Answer from the drawing. Dimensions are ordinates in mm from the lowest x, y and z of the part. Give positions to 0.01 mm unless a question says otherwise; leave off trailing zeros. Loops run counter-clockwise (first coordinate to the right, second up) from the corner with the lowest first, then second, coordinate; pieces in that order, holes last.
(1) Find section C-C, the plane y = 0.35. State how many separate pieces and enclosed holes the cut face has.
(2) Each of these flat-tipped pins is pushed along its axis until it touches: P1, Ø0.7, axis at x = 18.5, z = 3, coming from the -Y side; P2, Ø1.5, axis at x = 16.5, z = 2, coming from the -Y side. Where does it stop, or does it pass through?
(3) Find section B-B, the plane x = 18.5. Write down the section's boundary in (y, z).
(4) Find section D-D, the plane x = 7.75. Write down the section's boundary in (y, z) (1 decimal).
(5) Straight lines are drawn through the part: probe 1 along Z at (x, y) = (18.5, 0.3); probe 2 along Z at (x, y) = (3, 0.55). For each, find the intervals that lie inside material, in ascending order.
(6) Find section A-A, the plane z = 3. Write down the section's boundary in (x, y).
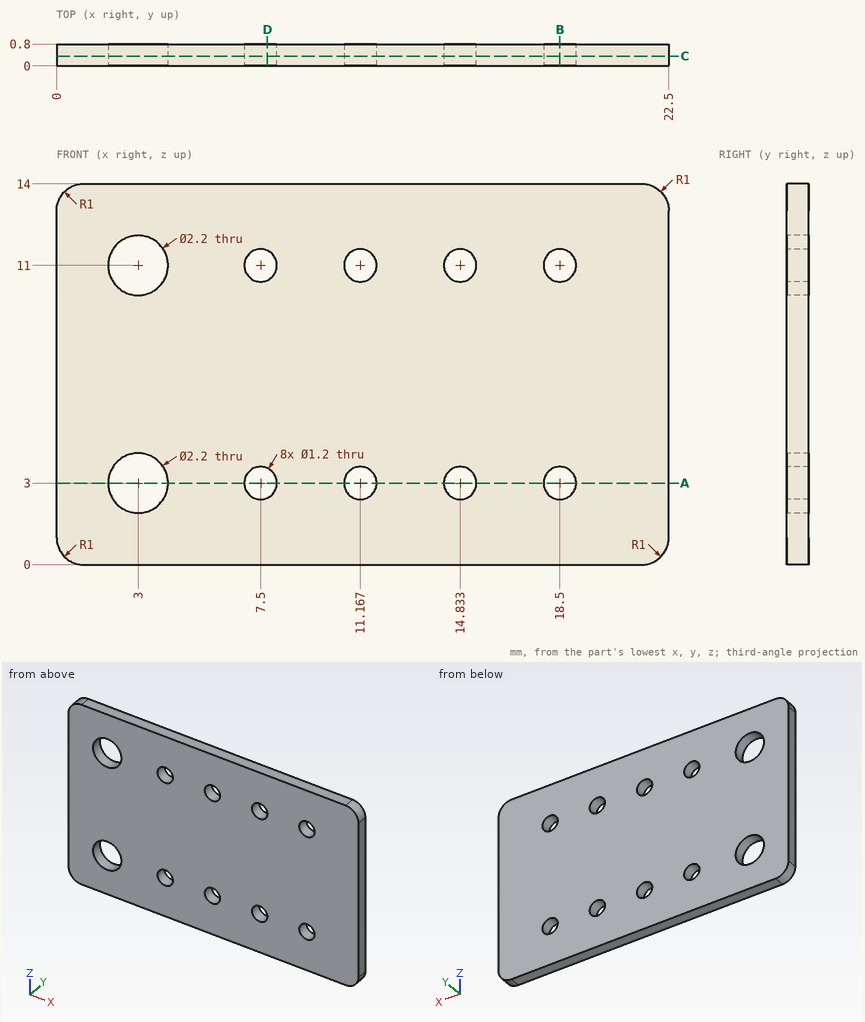
Entries:
1. separate pieces: 1
1. enclosed holes: 10
2. P1: passes through
2. P2: stops at y = 0
3. outline: (0, 0) - (0.8, 0) - (0.8, 2.4) - (0, 2.4) - close; (0, 3.6) - (0.8, 3.6) - (0.8, 10.4) - (0, 10.4) - close; (0, 11.6) - (0.8, 11.6) - (0.8, 14) - (0, 14) - close
4. outline: (0, 0) - (0.8, 0) - (0.8, 2.5) - (0, 2.5) - close; (0, 3.5) - (0.8, 3.5) - (0.8, 10.5) - (0, 10.5) - close; (0, 11.5) - (0.8, 11.5) - (0.8, 14) - (0, 14) - close
5. probe 1: z = 0 to 2.4, 3.6 to 10.4, 11.6 to 14
5. probe 2: z = 0 to 1.9, 4.1 to 9.9, 12.1 to 14
6. outline: (0, 0) - (1.9, 0) - (1.9, 0.8) - (0, 0.8) - close; (4.1, 0) - (6.9, 0) - (6.9, 0.8) - (4.1, 0.8) - close; (8.1, 0) - (10.57, 0) - (10.57, 0.8) - (8.1, 0.8) - close; (11.77, 0) - (14.23, 0) - (14.23, 0.8) - (11.77, 0.8) - close; (15.43, 0) - (17.9, 0) - (17.9, 0.8) - (15.43, 0.8) - close; (19.1, 0) - (22.5, 0) - (22.5, 0.8) - (19.1, 0.8) - close
